Could you check a few things on this model? Use its own coordinates, in mm. A direction names the side the tool comes from. Round coordinates to 2 decimals unless told otherwise and drop trailing zeros. Loops run counter-clockwise (first coordinate to the right, second up) from the corner with the lowest first, then second, coordinate; pieces in that order, holes last. Notation, with made-up numbers: M -2,12.5 L 32,12.5 A17 ccw 32,20.5 Z; hole C 24.25,21 d2. An arc over 180 degrees is marked long. One line per item, written item: value. Start each with the question number.
Q1. Which directions (+Z, -Z, +X, -X, +Y, -Y) give clear straight access to the entire face, cutting with the end or side of a thin tool? Please do faces 1 (the face through (10, 0, 5)), 2 (the face through (4.57, 7.167, 73.174)), 3 (the face through (-20.1, -1.6, 7)).
Q2. Please list where these lines run through material, in increasing order: line 1 along Y through (x, z) = (0, 51); line 2 along Z through (x, y) = (18, -11); line 3 along Z through (x, y) = (5.5, -7).
Q3. Imagine slicing it at D-D (x = 7). Please give me the cut outline in (y, z) (3 decimals).
Q4. I'm going to push flat-ended pins straight in: pin 1 Ø5 at (x, y) = (11.5, 8) entering from -Z; pin 2 Ø1.5 at (x, y) = (18, 9) entering from +Z; pin 3 Ø4 at (x, z) = (1.5, 35) entering from -Y. Where does each tip first touch, or does it pass through?
Q5. Imagine slicing it at C-C (z = 121). Please give me the cut outline in (x, y), then the cut area to 3 significant figures.
Q6. Thinking about a two-plate mould opening in Z: for faces 4 (the face through (10, 0, 15)), 5 (the face through (-4.336, -19.524, 9.958)), 6 (the face through (-20.1, -1.6, 13)), 7 (the face through (10.382, -19.961, 14.014)), which applies, released by +Z, released by -Z, zero draft, split by the parting line, or undercut?
Q7. Imagine slicing it at A-A (y = 0). Please give me the cut outline in (x, z), then the cut area to 3 significant figures.
from build123d import *

# Parameters (mm, degrees)
F0_R     = 8.5
F0_R_2   = 3
F1_DEPTH = 133
F0_R_3   = 20
F2_DEPTH = 15
F3_R     = 22.5
F4_DEPTH = 7
F3_R_2   = 20
F5_DEPTH = 5
F6_R     = 22.5
F6_R_2   = 20
F7_DEPTH = 2
F8_R     = 3
F9_DEPTH = 140


with BuildPart() as f1:
    # F0 (on Top) → F1 (new body)
    with BuildSketch(Plane.XY):
        Circle(F0_R)
        Circle(F0_R_2, mode=Mode.SUBTRACT)
    extrude(amount=F1_DEPTH)

    # F0 (on Top) → F2 (join)
    with BuildSketch(Plane.XY):
        Circle(F0_R_3)
        Circle(F0_R, mode=Mode.SUBTRACT)
    extrude(amount=F2_DEPTH)

    # F3 (on face) → F4 (join)
    with BuildSketch(Plane.XY):
        Circle(F3_R)
    extrude(amount=F4_DEPTH)

    # F3 (on face) + F0 (on Top) → F5 (cut)
    with BuildSketch(Plane.XY):
        Circle(F3_R)
        Circle(F3_R_2, mode=Mode.SUBTRACT)
    with BuildSketch(Plane.XY):
        Circle(F0_R_3)
        Circle(F0_R, mode=Mode.SUBTRACT)
    extrude(amount=F5_DEPTH, mode=Mode.SUBTRACT)

    # F6 (on face) → F7 (join)
    with BuildSketch(Plane.XY.offset(15)):
        Circle(F6_R)
        Circle(F6_R_2, mode=Mode.SUBTRACT)
    extrude(amount=-F7_DEPTH)

    # F8 (on face) → F9 (cut)
    with BuildSketch(Plane.XY):
        Circle(F8_R)
    extrude(amount=F9_DEPTH, mode=Mode.SUBTRACT)


solid = f1.part
Report:
1. face 1: -Z
1. face 2: +Z
1. face 3: none
2. line 1: y = -8.5 to -3, 3 to 8.5
2. line 2: z = 5 to 7, 13 to 15
2. line 3: z = 5 to 15
3. outline: M -21.383,5 L -4.822,5 L -4.822,0 L 4.822,0 L 4.822,5 L 21.383,5 L 21.383,7 L 18.735,7 L 18.735,13 L 21.383,13 L 21.383,15 L 4.822,15 L 4.822,133 L -4.822,133 L -4.822,15 L -21.383,15 L -21.383,13 L -18.735,13 L -18.735,7 L -21.383,7 Z
4. pin 1: stops at z = 5
4. pin 2: stops at z = 15
4. pin 3: stops at y = -8.5
5. outline: C 0,0 d17; hole C 0,0 d6
5. area: 199 mm²
6. face 4: released by +Z
6. face 5: undercut
6. face 6: undercut
6. face 7: zero draft
7. outline: M -22.5,5 L -8.5,5 L -8.5,0 L -3,0 L -3,133 L -8.5,133 L -8.5,15 L -22.5,15 L -22.5,13 L -20,13 L -20,7 L -22.5,7 Z; M 3,0 L 8.5,0 L 8.5,5 L 22.5,5 L 22.5,7 L 20,7 L 20,13 L 22.5,13 L 22.5,15 L 8.5,15 L 8.5,133 L 3,133 Z
7. area: 1,710 mm²
